```python
from build123d import *

# Parameters (mm, degrees)
F0_R     = 1.1684
F1_DEPTH = 4.5085
F3_DEPTH = 4.953
F5_DEPTH = 4.4069
F6_R     = 0.254
F7_DEPTH = 3.81


with BuildPart() as f1:
    # F0 (on Top) → F1 (new body, symmetric)
    with BuildSketch(Plane.XY):
        with BuildLine():
            Line((8.3947, 3.937), (-8.3947, 3.937))
            ThreePointArc((-8.3947, 3.937), (-9.508252, 3.475752), (-9.9695, 2.3622))
            Line((-9.9695, 2.3622), (-9.9695, -2.3622))
            ThreePointArc((-9.9695, -2.3622), (-9.508252, -3.475752), (-8.3947, -3.937))
            Line((-8.3947, -3.937), (8.3947, -3.937))
            ThreePointArc((8.3947, -3.937), (9.508252, -3.475752), (9.9695, -2.3622))
            Line((9.9695, -2.3622), (9.9695, 2.3622))
            ThreePointArc((9.9695, 2.3622), (9.508252, 3.475752), (8.3947, 3.937))
        make_face()
        with Locations((-7.1755, 0)):
            Circle(F0_R, mode=Mode.SUBTRACT)
        with Locations((7.1755, 0)):
            Circle(F0_R, mode=Mode.SUBTRACT)
    extrude(amount=F1_DEPTH, both=True)

    # F2 (on face) → F3 (join)
    with BuildSketch(Plane.XY.offset(4.5085)):
        with BuildLine():
            Line((-2.87642, -2.3622), (2.877878, -2.3622))
            ThreePointArc((2.877878, -2.3622), (4.234771, -1.586671), (4.255229, -0.023922))
            Line((4.255229, -0.023922), (3.396382, 1.525478))
            ThreePointArc((3.396382, 1.525478), (2.818303, 2.118894), (2.019031, 2.3368))
            Line((2.019031, 2.3368), (-2.017574, 2.3368))
            ThreePointArc((-2.017574, 2.3368), (-2.816845, 2.118894), (-3.394925, 1.525478))
            Line((-3.394925, 1.525478), (-4.253771, -0.023922))
            ThreePointArc((-4.253771, -0.023922), (-4.233314, -1.586671), (-2.87642, -2.3622))
        make_face()
    extrude(amount=F3_DEPTH)

    # F4 (on face) → F5 (join)
    with BuildSketch(Plane.XY.offset(9.4615)):
        with BuildLine():
            Line((1.832009, 2.0193), (-1.830552, 2.0193))
            ThreePointArc((-1.830552, 2.0193), (-2.629823, 1.801394), (-3.207903, 1.207978))
            Line((-3.207903, 1.207978), (-3.965627, -0.158992))
            ThreePointArc((-3.965627, -0.158992), (-3.949129, -1.419274), (-2.85486, -2.0447))
            Line((-2.85486, -2.0447), (2.856317, -2.0447))
            ThreePointArc((2.856317, -2.0447), (3.950586, -1.419274), (3.967084, -0.158992))
            Line((3.967084, -0.158992), (3.209361, 1.207978))
            ThreePointArc((3.209361, 1.207978), (2.631281, 1.801394), (1.832009, 2.0193))
        make_face()
    extrude(amount=F5_DEPTH)

    # F6 (on face) → F7 (join)
    with BuildSketch(Plane(origin=(0, 0, -4.5085), x_dir=(1, 0, 0), z_dir=(0, 0, -1))):
        with Locations((-3.7973, 0.9525)):
            Circle(F6_R)
        with Locations((-1.8923, 0.9525)):
            Circle(F6_R)
        with Locations((0.0127, 0.9525)):
            Circle(F6_R)
        with Locations((1.9177, 0.9525)):
            Circle(F6_R)
        with Locations((3.8227, 0.9525)):
            Circle(F6_R)
        with Locations((-2.8448, -0.9525)):
            Circle(F6_R)
        with Locations((-0.9398, -0.9525)):
            Circle(F6_R)
        with Locations((0.9652, -0.9525)):
            Circle(F6_R)
        with Locations((2.8702, -0.9525)):
            Circle(F6_R)
    extrude(amount=F7_DEPTH)


solid = f1.part
```
Build history of the part. All positions in model axes, mm. A direction names the side the tool comes from. Give positions to 0.01 mm unless a question says otherwise; leave off trailing zeros. Order: outer loops, then holes, each group sorted by start corner. A loop starts at its lowest first (then second) coordinate and runs counter-clockwise, first axis right, second up. Notation, with made-up numbers: M 2.25,26.5 L 29.25,26.5 A9 ccw 29.25,41.5 Z; hole C -37.5,54 d2. An arc over 180 degrees is marked long. Write item = value, one per line. Start each with the question number.
(1) Which spindle directions (+Z, -Z, +X, -X, +Y, -Y) get a long thin tool onto all of the face, cutting with end or side? Do faces 1 (the cylindrical face through (3.94, -1.44, 11.63)), 2 (the flat face through (3.83, 0.74, 6.95)), 3 (the flat face through (0, 3, 4.508)), 4 (the cylindrical face through (-4.245, -1.567, 6.95)). Say none if no direction does.
(2) Slice it at B-B on z = 6.25. Write the cut outline in (x, y), plus the area to 3 significant figures.
(3) Slice it at A-A on z = -5.25. State how many separate pieces and enclosed holes the cut face has, plus the area to 3 significant figures.
(4) Slice it at C-C on x = 7.5. Write the cut outline in (y, z), plus the area to 3 significant figures.
(5) Probe L1, parallel to Z at x = -0.5, y = -0.5; L2, parallel to Z at x = 2, y = 3.75; L3, parallel to Y at x = -6.5, z = 3. List the from-to ranges inside material, lowest first. Write a range as [from, to].
(6) Slice it at D-D on y = -1.5. Write the cut outline in (x, z), plus the area to 3 significant figures.
(7) Pin check, flat tips, straight feed: pin 1 Ø4 at (x, y) = (6, -3) entering from -Z; pin 2 Ø4 at (x, z) = (-0.5, 11) entering from +Y; pin 3 Ø2.5 at (x, y) = (3, -0.5) entering from -Z; pin 4 Ø2 at (x, y) = (7.18, 0) entering from -Z. Stop position of each tip, or through.
Responses:
q1.face_1 = +Z, +X
q1.face_2 = +Z, +X, +Y
q1.face_3 = +Z
q1.face_4 = +Z, -X
q2.outline = M -4.25,-0.02 A1.57 ccw -2.88,-2.36 L 2.88,-2.36 A1.57 ccw 4.26,-0.02 L 3.4,1.53 A1.57 ccw 2.02,2.34 L -2.02,2.34 A1.57 ccw -3.39,1.53 Z
q2.area = 36.4 mm2
q3.separate_pieces = 9
q3.enclosed_holes = 0
q3.area = 1.82 mm2
q4.outline = M -3.94,-4.51 L -1.12,-4.51 L -1.12,4.51 L -3.94,4.51 Z; M 1.12,-4.51 L 3.94,-4.51 L 3.94,4.51 L 1.12,4.51 Z
q4.area = 50.8 mm2
q5.L1 = [-4.51, 13.87]
q5.L2 = [-4.51, 4.51]
q5.L3 = [-3.94, -0.95], [0.95, 3.94]
q6.outline = M -9.97,-4.51 L 9.97,-4.51 L 9.97,4.51 L 4.28,4.51 L 4.28,9.46 L 3.9,9.46 L 3.9,13.87 L -3.9,13.87 L -3.9,9.46 L -4.28,9.46 L -4.28,4.51 L -9.97,4.51 Z
q6.area = 257 mm2
q7.pin_1 = -4.51
q7.pin_2 = 2.34
q7.pin_3 = -8.32
q7.pin_4 = through
